Build history of the part. All positions in model axes, mm. Face numbers are marked on the shaded views. A direction names the side the tool comes from. Give positions to 0.01 mm unless a question says otherwise; leave off trailing zeros. Order: outer loops, then holes, each group sorted by start corner. A loop starts at its lowest first (then second) coordinate and runs counter-clockwise, first axis right, second up. Notation, with made-up numbers: (-10.75, 64) - (13.25, 64) arc R14 cw to (13.25, 91) - close; hole circle Ø2 at (-0.75, -19). An arc over 180 degrees is marked (long way). One line per item, written item: value.
```python
from build123d import *

# Parameters (mm, degrees)
F0_W      = 58
F0_H      = 58
F0_R      = 2.25
F1_DEPTH  = 7
F3_DEPTH  = 30
F4_R      = 2.25
F5_DEPTH  = 25
F6_R      = 2.25
F7_DEPTH  = 25
F8_R      = 1
F9_R      = 1
F10_R     = 1
F11_R     = 1
F12_SIZE2 = 2.25
F12_SIZE  = 2.25
F13_W     = 1.5
F13_H     = 22
F14_DEPTH = 4
F15_W     = 1.5
F15_H     = 22
F16_DEPTH = 4
F17_R     = 0.5
F18_R     = 0.5


with BuildPart() as f1:
    # F0 (on Top) → F1 (new body)
    with BuildSketch(Plane.XY):
        with Locations((-29, 29)):
            Rectangle(F0_W, F0_H)
        with Locations((-33, 33)):
            Circle(F0_R, mode=Mode.SUBTRACT)
    extrude(amount=F1_DEPTH)

    # F2 (on face) → F3 (join)
    with BuildSketch(Plane(origin=(0, 0, 0), x_dir=(1, 0, 0), z_dir=(0, 0, -1))):
        Polygon((0, -58), (0, 0), (-58, 0), (-58, -7), (-7, -7), (-7, -58), align=None)
    extrude(amount=F3_DEPTH)

    # F4 (on face) → F5 (cut)
    with BuildSketch(Plane(origin=(-7, 0, 0), x_dir=(0, -1, 0), z_dir=(-1, 0, 0))):
        with Locations((-32.6, -15)):
            Circle(F4_R)
    extrude(amount=-F5_DEPTH, mode=Mode.SUBTRACT)

    # F6 (on face) → F7 (cut)
    with BuildSketch(Plane(origin=(0, 7, 0), x_dir=(-1, 0, 0), z_dir=(0, 1, 0))):
        with Locations((32.6, -15)):
            Circle(F6_R)
    extrude(amount=-F7_DEPTH, mode=Mode.SUBTRACT)

    # F8
    f8_edges = [f1.edges().sort_by_distance(p)[0] for p in [
        (-29, 0, -30),
    ]]
    fillet(f8_edges, radius=F8_R)

    # F9
    f9_edges = [f1.edges().sort_by_distance(p)[0] for p in [
        (0, 29.5, -30),
    ]]
    fillet(f9_edges, radius=F9_R)

    # F10
    f10_edges = [f1.edges().sort_by_distance(p)[0] for p in [
        (-7, 32.5, 0),
        (-7, 7, -15),
        (-32.5, 7, 0),
    ]]
    fillet(f10_edges, radius=F10_R)

    # F11
    f11_edges = [f1.edges().sort_by_distance(p)[0] for p in [
        (-58, 4, -30),
        (-58, 0, -11),
        (-58, 33, 0),
        (-58, 7, -15.5),
        (-58, 7.292893, -0.292893),
        (-58, 0.292893, -29.707107),
        (-58, 58, 3.5),
        (-33, 58, 0),
        (-7.292893, 58, -0.292893),
        (-4, 58, -30),
        (-7, 58, -15.5),
        (0, 58, -11),
    ]]
    fillet(f11_edges, radius=F11_R)

    # F12
    f12_edges = [f1.edges().sort_by_distance(p)[0] for p in [
        (-35.25, 33, 0),
        (-30.35, 0, -15),
        (0, 34.85, -15),
    ]]
    chamfer(f12_edges, length=F12_SIZE, length2=F12_SIZE2)

    # F13 (on face) → F14 (join)
    with BuildSketch(Plane.XZ):
        with Locations((-50.65, -4)):
            Rectangle(F13_W, F13_H)
        with Locations((-54.25, -4)):
            Rectangle(F13_W, F13_H)
    extrude(amount=F14_DEPTH)

    # F15 (on face) → F16 (join)
    with BuildSketch(Plane.YZ):
        with Locations((54.25, -4)):
            Rectangle(F15_W, F15_H)
        with Locations((50.65, -4)):
            Rectangle(F15_W, F15_H)
    extrude(amount=F16_DEPTH)

    # F17
    f17_edges = [f1.edges().sort_by_distance(p)[0] for p in [
        (4, 54.25, -15),
        (4, 50.65, -15),
        (2, 51.4, -15),
        (2, 49.9, -15),
        (4, 49.9, -4),
        (2, 53.5, -15),
        (2, 55, -15),
        (4, 55, -4),
    ]]
    fillet(f17_edges, radius=F17_R)

    # F18
    f18_edges = [f1.edges().sort_by_distance(p)[0] for p in [
        (-50.65, -4, -15),
        (-54.25, -4, -15),
        (-49.9, -4, -4),
        (-49.9, -2, -15),
        (-55, -4, -4),
        (-55, -2, -15),
        (-53.5, -2, -15),
        (-51.4, -2, -15),
    ]]
    fillet(f18_edges, radius=F18_R)


solid = f1.part
```
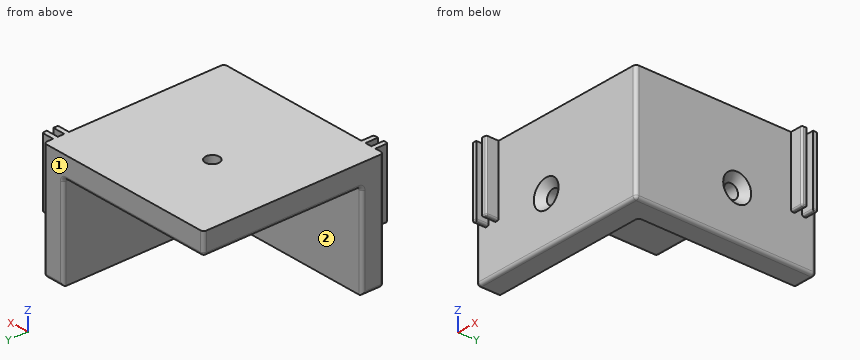
(1) 3-axis set-ups, long thin cutter, end or side, ignore diameter. For the marked faces 1 and 2: which of +Z, -Z, +X, -X, +Y, -Y reach the whole face in a straight line?
Completed:
face 1: +Z, -Z, +X, -X, +Y
face 2: -Z, -X, +Y
(2) Slice it at B-B, the plane z = -20.5. Give the cut face in (x, y), and give its area (3 significant figures).
Completed:
outline: (-58, 1) arc R1 ccw to (-57, 0) - (-1, 0) arc R1 ccw to (0, 1) - (0, 57) arc R1 ccw to (-1, 58) - (-6, 58) arc R1 ccw to (-7, 57) - (-7, 8) arc R1 cw to (-8, 7) - (-57, 7) arc R1 ccw to (-58, 6) - close
area: 762 mm²
(3) Slice it at C-C, the plane y = 33. Count the separate pieces of the cut face and the enclosed holes in it, and give its area (3 significant figures).
Completed:
separate pieces: 3
enclosed holes: 0
area: 543 mm²
(4) Pin check, flat tips, straight feed: P1, Ø4, axis at x = 2.5, z = -6, coming from the -Y side; P2, Ø12, axis at x = -41.5, y = 10, coming from the -Z side; P3, Ø1.2, axis at x = 2.5, z = -7, coming from the +Y side; P4, Ø1, axis at x = -35, y = 36.5, coming from the -Z side. Stop position of each tip, or through.
Completed:
P1: y = 49.9
P2: z = -30
P3: y = 55
P4: z = 0
(5) Drill centre lines: line 1 (Y direction, x = -33, z = 5.35); line 2 (Z direction, x = -32.6, y = 3.6); line 3 (Y direction, x = -15, z = 2.5). Where is each one in solid material? Low to high.
Completed:
line 1: 0 to 30.75, 35.25 to 58
line 2: -30 to -17.25, -12.75 to 7
line 3: 0 to 58
(6) Slice it at A-A, the plane x = -39. Give the cut face in (y, z), and give its area (3 significant figures).
Completed:
outline: (0, -29) arc R1 ccw to (1, -30) - (7, -30) - (7, -1) arc R1 cw to (8, 0) - (57, 0) arc R1 ccw to (58, 1) - (58, 7) - (0, 7) - close
area: 616 mm²
